Source: CAD feature listing. Evaluate the final solid. Frame: model axes, mm. Face numbers are marked on the shaded views. Coordinates: 2 decimals unless noted, no trailing zeros. Loops run counter-clockwise (first coordinate to the right, second up) from the corner with the lowest first, then second, coordinate; pieces in that order, holes last.
Item 1: Pull-direction query (X, two-part tool) for the marked faces 1, 2, 3 and 4; classes: +X half, -X half, draft (parallel to the pull), parting line (faces both ways), or undercut.
Item 2: Pin query (flat end, axial travel): pin 1 Ø4 at (x, y) = (13.5, 3) entering from -Z; pin 2 Ø1.5 at (x, y) = (6, 2) entering from +Z; pin 3 Ø3.5 at (x, z) = (0, -35.5) entering from -Y; pin 4 Ø1.5 at (y, z) = (4.5, -6) entering from +X. Return the tip coordinate at first contact, or that it passes through.
Item 3: Section query D-D, the plane z = -10. Return the cut outline in (x, y).
Item 4: Section query C-C, the plane y = 3.5. Return the cut outline in (x, z), then the cut area to 3 significant figures.
Item 5: Section query B-B, the plane x = 0. Return the cut outline in (y, z).
Item 6: Section query A-A, the plane z = 0. Return the cut outline in (x, y), then the cut area to 3 significant figures.
Item 7: Line query: probe 1 along X at (y, z) = (0.5, 9.5); probe 2 along X at (y, z) = (6.75, -7); probe 3 along Z at (x, y) = (-15, 2.5). Output: solid intervals per line, ascending.
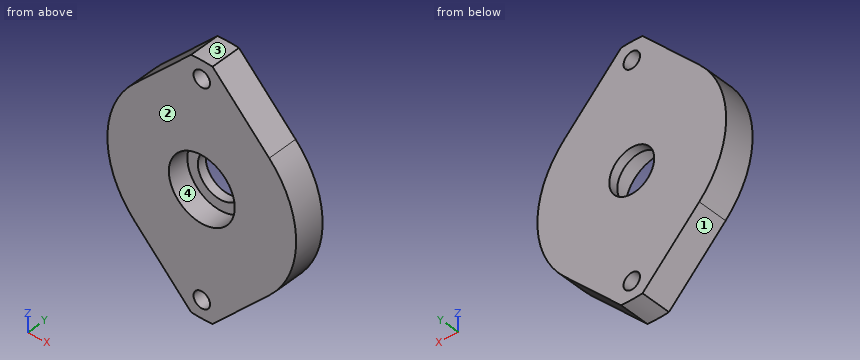
```python
from build123d import *

# Parameters (mm, degrees)
SKETCH1_R            = 41.5
BOSS_EXTRUDE1_DEPTH  = 10
SKETCH2_OUTSIDE_W    = 108.56
SKETCH2_OUTSIDE_H    = 108.56
CUT_EXTRUDE1_DEPTH   = 10
SKETCH3_R            = 11
CUT_EXTRUDE2_DEPTH   = 7
CUT_EXTRUDE3_REACH   = 54.569
SKETCH4_R            = 7.5
M5_CLEARANCE_HOLE1_D = 5.5


with BuildPart() as part:
    # Sketch1 → Boss-Extrude1 (new body)
    with BuildSketch(Plane(origin=(0, 0, 0), x_dir=(1, 0, 0), z_dir=(0, 1, 0))):
        with Locations(Location((0, 0, 0), (0, 0, 270))):
            Circle(SKETCH1_R)
    extrude(amount=BOSS_EXTRUDE1_DEPTH)

    # Sketch2 outside → Cut-Extrude1 (cut)
    with BuildSketch(Plane.XZ):
        Rectangle(SKETCH2_OUTSIDE_W, SKETCH2_OUTSIDE_H)
        with BuildLine():
            Line((-22.5, 22.045407685), (-3.590980448, 41.344344951))
            ThreePointArc((-3.590980448, 41.344344951), (0, 41.5), (3.590980448, 41.344344951))
            Line((3.590980448, 41.344344951), (22.5, 22.045407685))
            ThreePointArc((22.5, 22.045407685), (31.5, 0), (22.5, -22.045407685))
            Line((22.5, -22.045407685), (3.590980448, -41.344344951))
            ThreePointArc((3.590980448, -41.344344951), (0, -41.5), (-3.590980448, -41.344344951))
            Line((-3.590980448, -41.344344951), (-22.5, -22.045407685))
            ThreePointArc((-22.5, -22.045407685), (-31.5, 0), (-22.5, 22.045407685))
        make_face(mode=Mode.SUBTRACT)
    extrude(amount=-CUT_EXTRUDE1_DEPTH, mode=Mode.SUBTRACT)

    # Sketch3 → Cut-Extrude2 (cut)
    with BuildSketch(Plane(origin=(0, 0, 0), x_dir=(1, 0, 0), z_dir=(0, 1, 0))):
        with Locations(Location((0, 0, 0), (0, 0, 270))):
            Circle(SKETCH3_R)
    extrude(amount=CUT_EXTRUDE2_DEPTH, mode=Mode.SUBTRACT)

    # Sketch4 → Cut-Extrude3 (cut, up to next)
    with BuildSketch(Plane.XZ.offset(-7), mode=Mode.PRIVATE) as cut_extrude3_sk1:
        with Locations(Location((0, 0, 0), (0, 0, 270))):
            Circle(SKETCH4_R)
    cut_extrude3_tool1 = extrude(cut_extrude3_sk1.sketch, amount=-CUT_EXTRUDE3_REACH, mode=Mode.PRIVATE) & part.part
    add(cut_extrude3_tool1.solids().sort_by_distance((0, 7, 0))[0], mode=Mode.SUBTRACT)

    # M5 Clearance Hole1 (through all)
    with Locations(Plane(origin=(0, 0, 0), x_dir=(-1, 0, 0), z_dir=(0, -1, 0))):
        with Locations((0, 35.5), (0, -35.5)):
            Hole(M5_CLEARANCE_HOLE1_D / 2)


solid = part.part
```
Verdict:
1. face 1: -X half
1. face 2: draft
1. face 3: parting line
1. face 4: undercut
2. pin 1: stops at z = -33.27
2. pin 2: stops at z = 39.65
2. pin 3: passes through
2. pin 4: stops at x = 31.06
3. outline: (-29.87, 0) - (-4.58, 0) - (-4.58, 7) - (4.58, 7) - (4.58, 0) - (29.87, 0) - (29.87, 10) - (-29.87, 10) - close
4. outline: (-22.5, -22.05) - (-3.59, -41.34) arc R41.5 ccw to (3.59, -41.34) - (22.5, -22.05) arc R31.5 ccw to (22.5, 22.05) - (3.59, 41.34) arc R41.5 ccw to (-3.59, 41.34) - (-22.5, 22.05) arc R31.5 ccw to start; hole circle Ø22 at (0, 0); hole circle Ø5.5 at (0, -35.5); hole circle Ø5.5 at (0, 35.5)
4. area: 3,110 mm2
5. outline: (0, -41.5) - (10, -41.5) - (10, -38.25) - (0, -38.25) - close; (0, -32.75) - (10, -32.75) - (10, -7.5) - (7, -7.5) - (7, -11) - (0, -11) - close; (0, 11) - (7, 11) - (7, 7.5) - (10, 7.5) - (10, 32.75) - (0, 32.75) - close; (0, 38.25) - (10, 38.25) - (10, 41.5) - (0, 41.5) - close
6. outline: (-31.5, 0) - (-11, 0) - (-11, 7) - (-7.5, 7) - (-7.5, 10) - (-31.5, 10) - close; (7.5, 7) - (11, 7) - (11, 0) - (31.5, 0) - (31.5, 10) - (7.5, 10) - close
6. area: 431 mm2
7. probe 1: x = -30.03 to -5.55, 5.55 to 30.03
7. probe 2: x = -30.71 to -8.49, 8.49 to 30.71
7. probe 3: z = -29.7 to 29.7
